Source: CAD feature listing. Evaluate the final solid. Frame: model axes, mm. Face numbers are marked on the shaded views. A direction names the side the tool comes from. Round coordinates to 2 decimals unless told otherwise and drop trailing zeros. Write each loop counter-clockwise with the first axis right and the second up, starting at its lowest first coordinate (ties: lowest second). Pieces come first, ordered by that corner, then holes. Notation, with made-up numbers: (86.5, 29) -> (121.5, 29) arc R21 cw to (121.5, 57) -> close; hole circle Ø5 at (48.5, 74.5). An arc over 180 degrees is marked (long way). Put each result on its own line as item: value.
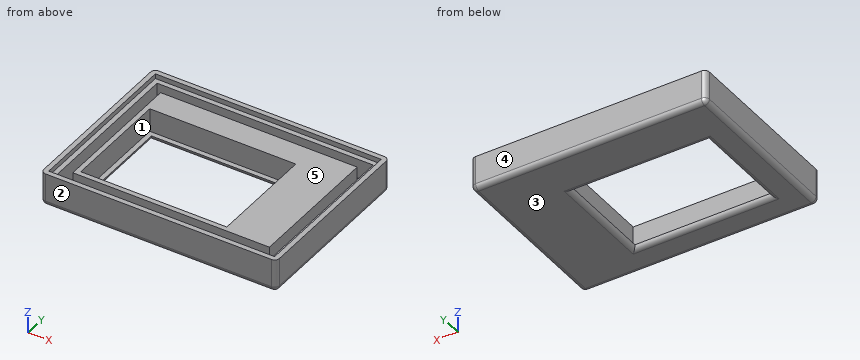
```python
from build123d import *

# Parameters (mm, degrees)
F0_W     = 242
F0_H     = 180
F1_DEPTH = 34
F2_W     = 140
F2_H     = 100
F3_DEPTH = 34.001
F4_W     = 150
F4_H     = 110
F4_W_2   = 140
F4_H_2   = 100
F5_DEPTH = 29
F6_W     = 232
F6_H     = 170
F6_W_2   = 150
F6_H_2   = 110
F7_DEPTH = 5
F8_W     = 222
F8_H     = 160
F8_W_2   = 202
F8_H_2   = 140
F9_DEPTH = 20
F10_R    = 5
F11_R    = 4.99999


# Not quite as in the source:
# - a fillet or chamfer is up to 0.001 mm smaller than in the source, because OpenCascade refuses the exact size


with BuildPart() as f1:
    # F0 (on Top) → F1 (new body)
    with BuildSketch(Plane.XY):
        with Locations((121, 90)):
            Rectangle(F0_W, F0_H)
    extrude(amount=F1_DEPTH)

    # F2 (on face) → F3 (cut, through all)
    with BuildSketch(Plane.XY.offset(34)):
        with Locations((100, 80)):
            Rectangle(F2_W, F2_H)
    extrude(amount=-F3_DEPTH, mode=Mode.SUBTRACT)

    # F4 (on face) → F5 (cut)
    with BuildSketch(Plane.XY.offset(34)):
        with Locations((100, 80)):
            Rectangle(F4_W, F4_H)
        with Locations((100, 80)):
            Rectangle(F4_W_2, F4_H_2, mode=Mode.SUBTRACT)
    extrude(amount=-F5_DEPTH, mode=Mode.SUBTRACT)

    # F6 (on face) → F7 (cut)
    with BuildSketch(Plane.XY.offset(34)):
        with Locations((121, 90)):
            Rectangle(F6_W, F6_H)
        with Locations((100, 80)):
            Rectangle(F6_W_2, F6_H_2, mode=Mode.SUBTRACT)
    extrude(amount=-F7_DEPTH, mode=Mode.SUBTRACT)

    # F8 (on face) → F9 (cut)
    with BuildSketch(Plane.XY.offset(29)):
        with Locations((121, 90)):
            Rectangle(F8_W, F8_H)
        with Locations((121, 90)):
            Rectangle(F8_W_2, F8_H_2, mode=Mode.SUBTRACT)
    extrude(amount=-F9_DEPTH, mode=Mode.SUBTRACT)

    # F10
    f10_edges = [f1.edges().sort_by_distance(p)[0] for p in [
        (242, 0, 17),
        (242, 180, 17),
        (0, 180, 17),
        (0, 0, 17),
    ]]
    fillet(f10_edges, radius=F10_R)

    # F11 (radius 5 in the source; OpenCascade refuses exactly that, so slightly less here)
    f11_edges = [f1.edges().sort_by_distance(p)[0] for p in [
        (121, 0, 0),
        (170, 80, 0),
        (100, 30, 0),
        (30, 80, 0),
        (100, 130, 0),
    ]]
    fillet(f11_edges, radius=F11_R)


solid = f1.part
```
Q1. Cut plane B-B on z = 12.5. Output: boundary loops of the cut face in (x, y), and give its area (3 significant figures).
Ans:
outline: (0, 5) arc R5 ccw to (5, 0) -> (237, 0) arc R5 ccw to (242, 5) -> (242, 175) arc R5 ccw to (237, 180) -> (5, 180) arc R5 ccw to (0, 175) -> close; (20, 20) -> (222, 20) -> (222, 160) -> (20, 160) -> close; hole (10, 10) -> (232, 10) -> (232, 170) -> (10, 170) -> close; hole (25, 25) -> (175, 25) -> (175, 135) -> (25, 135) -> close
area: 19,800 mm^2
Q2. Reachability of the marked faces 4 and 5 from +Z, -Z, +X, -X, +Y, -Y: full face, straight path, thin tool, end or side. Return the list, or none.
Ans:
face 4: +Z, -Z, +X, -X, +Y
face 5: +Z
Q3. Material intervals for line 1 (Y direction, x = 160.5, z = 10.5); line 2 (X direction, y = 142.5, z = 20.5); line 3 (X direction, y = 88.5, z = 11), sorted ascending. Write a range as [from, to].
Ans:
line 1: y = [0, 10], [20, 25], [135, 160], [170, 180]
line 2: x = [0, 10], [20, 222], [232, 242]
line 3: x = [0, 10], [20, 25], [175, 222], [232, 242]
Q4. Pin query (flat end, axial travel): pin 1 (4 mm diameter, centred on x = 37, y = 149, fed in from +Z). Return the tip coordinate at first contact, or that it passes through.
Ans:
pin 1: stops at z = 29
Q5. Draft query along Y for the marked faces 1, 2 and 3. Return one class per face: +Y half, -Y half, draft (parallel to the pull), parting line (faces both ways), or undercut.
Ans:
face 1: undercut
face 2: -Y half
face 3: draft
Q6. Cut plane D-D on x = 190. Output: boundary loops of the cut face in (y, z).
Ans:
outline: (0, 5) arc R5 ccw to (5, 0) -> (175, 0) arc R5 ccw to (180, 5) -> (180, 34) -> (175, 34) -> (175, 29) -> (170, 29) -> (170, 9) -> (160, 9) -> (160, 29) -> (20, 29) -> (20, 9) -> (10, 9) -> (10, 29) -> (5, 29) -> (5, 34) -> (0, 34) -> close
